from build123d import *

# Parameters (mm, degrees)
F1_DEPTH = 5
F2_W     = 600
F2_H     = 5
F3_DEPTH = 80
F4_W     = 600
F4_H     = 5
F4_H_2   = 195
F5_DEPTH = 5
F6_R     = 10
F7_R     = 4
F8_DEPTH = 85


# Not quite as in the source:
# - a feature names something its author has since deleted; it is built from what else it names


with BuildPart() as f1:
    # F0 (on Front) → F1 (new body)
    with BuildSketch(Plane.XZ):
        with BuildLine():
            Line((26.5459360182, 400.2749490738), (-553.4540639818, 400.2749490738))
            ThreePointArc((-553.4540639818, 400.2749490738), (-560.5251317936, 397.3460168857), (-563.4540639818, 390.2749490738))
            Line((-563.4540639818, 390.2749490738), (-563.4540639818, -19.7250509262))
            Line((-563.4540639818, -19.7250509262), (36.5459360182, -19.7250509262))
            Line((36.5459360182, -19.7250509262), (36.5459360182, 390.2749490738))
            ThreePointArc((36.5459360182, 390.2749490738), (33.6170038301, 397.3460168857), (26.5459360182, 400.2749490738))
        make_face()
    extrude(amount=F1_DEPTH)

    # F2 (on face) → F3 (join)
    with BuildSketch(Plane.XZ.offset(5)):
        with Locations((-263.4540639818, -17.2250509262)):
            Rectangle(F2_W, F2_H)
    extrude(amount=F3_DEPTH)

    # F4 (on face) → F5 (join)
    with BuildSketch(Plane.XZ.offset(85)):
        with Locations((-263.4540639818, -17.2250509262)):
            Rectangle(F4_W, F4_H)
        with Locations((-263.4540639818, 82.7749490738)):
            Rectangle(F4_W, F4_H_2)
    extrude(amount=F5_DEPTH)

    # F6
    f6_edges = [f1.edges().sort_by_distance(p)[0] for p in [
        (-563.454064, -87.5, 180.274949),
        (36.545936, -87.5, 180.274949),
    ]]
    fillet(f6_edges, radius=F6_R)

    # F7 (on face) → F8 (join)
    with BuildSketch(Plane.XZ.offset(90)):
        with Locations((-543.4540639818, 161.7681980133)):
            Circle(F7_R)
        with Locations((16.5459360182, 161.7681980133)):
            Circle(F7_R)
    extrude(amount=-F8_DEPTH)


solid = f1.part
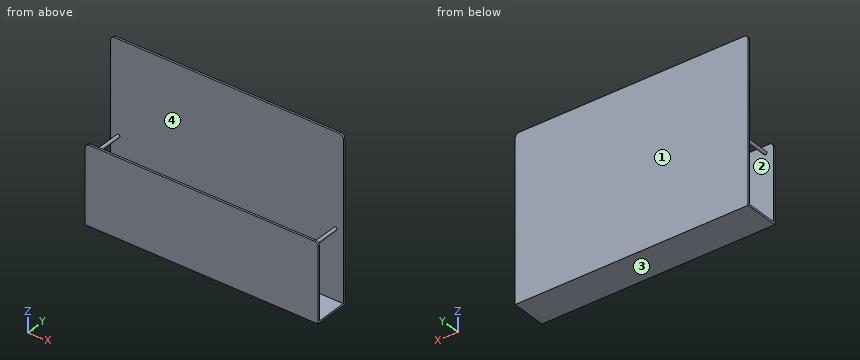
Verification items for the finished model (mm, model axes). Face numbers are marked on the shaded views. Round coordinates to 2 decimals unless told otherwise and drop trailing zeros. Order: outer loops, then holes, each group sorted by start corner. A loop starts at its lowest first (then second) coordinate and runs counter-clockwise, first axis right, second up.
1. Thickness scan on L1, parallel to Y at x = -232, z = 15.5; L2, parallel to Z at x = -38.5, y = -10; L3, parallel to Y at x = -475, z = 380.5. Record the ranges inside material, lowest first.
Final values:
L1: y = -90 to -85, -5 to 0
L2: z = -19.73 to -14.73
L3: y = -5 to 0
2. Go/stop test with flat-tipped pins: P1, Ø8, axis at x = -294.5, y = -29.5, coming from the +Z side; P2, Ø4, axis at x = -224.5, y = -87.5, coming from the +Z side. Record where each tip stops, or that it passes through.
Final values:
P1: stops at z = -14.73
P2: stops at z = 180.27
3. Release check for a two-part mould opening along Y. For the marked faces 1, 2, 3 and 4 record: +Y half, -Y half, draft (parallel to the pull), parting line (faces both ways), or undercut.
Final values:
face 1: +Y half
face 2: undercut
face 3: draft
face 4: undercut
4. Section check D-D on z = 201. Record the cut outline in (x, y), then the cut area to 3 significant figures.
Final values:
outline: (-563.45, -5) - (36.55, -5) - (36.55, 0) - (-563.45, 0) - close
area: 3,000 mm2
5. Section check C-C on x = -194. Record the cut outline in (y, z).
Final values:
outline: (-90, -19.73) - (0, -19.73) - (0, 400.27) - (-5, 400.27) - (-5, -14.73) - (-85, -14.73) - (-85, 180.27) - (-90, 180.27) - close
6. Section check B-B on y = -38.5. Record the cut outline in (x, z), then the cut area to 3 significant figures.
Final values:
outline: (-563.45, -19.73) - (36.55, -19.73) - (36.55, -14.73) - (-563.45, -14.73) - close; circle Ø8 at (-543.45, 161.77); circle Ø8 at (16.55, 161.77)
area: 3,100 mm2
7. Section check A-A on z = 48.5. Record the cut outline in (x, y).
Final values:
outline: (-563.45, -90) - (36.55, -90) - (36.55, -85) - (-563.45, -85) - close; (-563.45, -5) - (36.55, -5) - (36.55, 0) - (-563.45, 0) - close
